The figure shows three views and two pictorial views of one solid part (mm, origin at its lowest corner). Answer the questions. Give positions to 0.01 mm unless a question says otherwise; leave off trailing zeros. Loops run counter-clockwise (first coordinate to the right, second up) from the corner with the lowest first, then second, coordinate; pieces in that order, holes last. Notation, with made-up numbers: M -13,76 L 21,76 A26 ccw 21,111 Z; hole C 62,41.25 d7. An arc over 180 degrees is marked long. Answer in a Markdown table with one row per item. Add a question column.
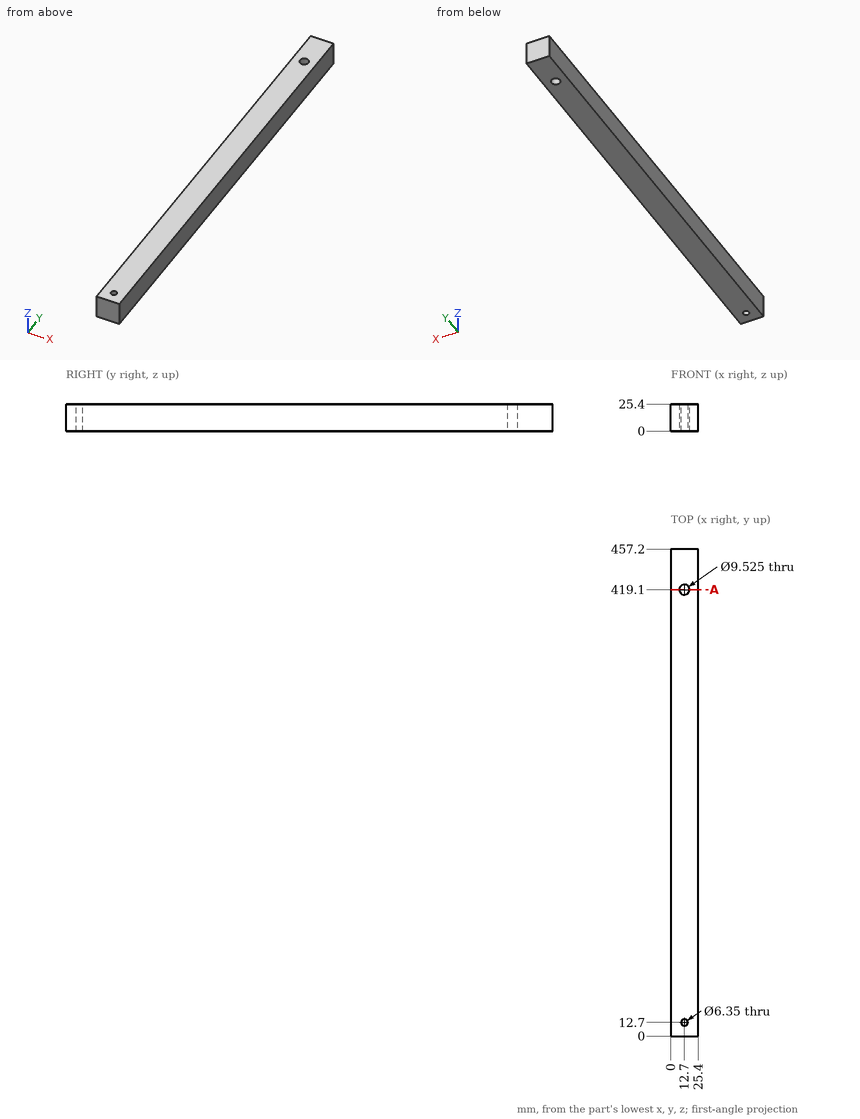
(1) Section A-A, the plane y = 419.1 is taken. Determine the outline of the cut face in (x, z), and give its area (3 significant figures).
(2) This flat-tipped pin is pushed along its axis until it touches: P1, Ø10, axis at x = 12.7, y = 12.7, coming from the +Z side. Where does it stop, or does it pass through?
(3) Consider line 1 along Y through (x, z) = (12.5, 18.25); line 2 along Y through (x, z) = (11.5, 14); line 3 along X through (y, z) = (419.1, 16.5). Determine where each line is inside the solid, lowest interval first. Write a range as from..to.
Numbers:
| question | item | result |
|---|---|---|
| 1 | outline | M 0,0 L 7.94,0 L 7.94,25.4 L 0,25.4 Z; M 17.46,0 L 25.4,0 L 25.4,25.4 L 17.46,25.4 Z |
| 1 | area | 403 mm² |
| 2 | P1 | stops at z = 25.4 |
| 3 | line 1 | y = 0..9.53, 15.87..414.34, 423.86..457.2 |
| 3 | line 2 | y = 0..9.76, 15.64..414.49, 423.71..457.2 |
| 3 | line 3 | x = 0..7.94, 17.46..25.4 |
